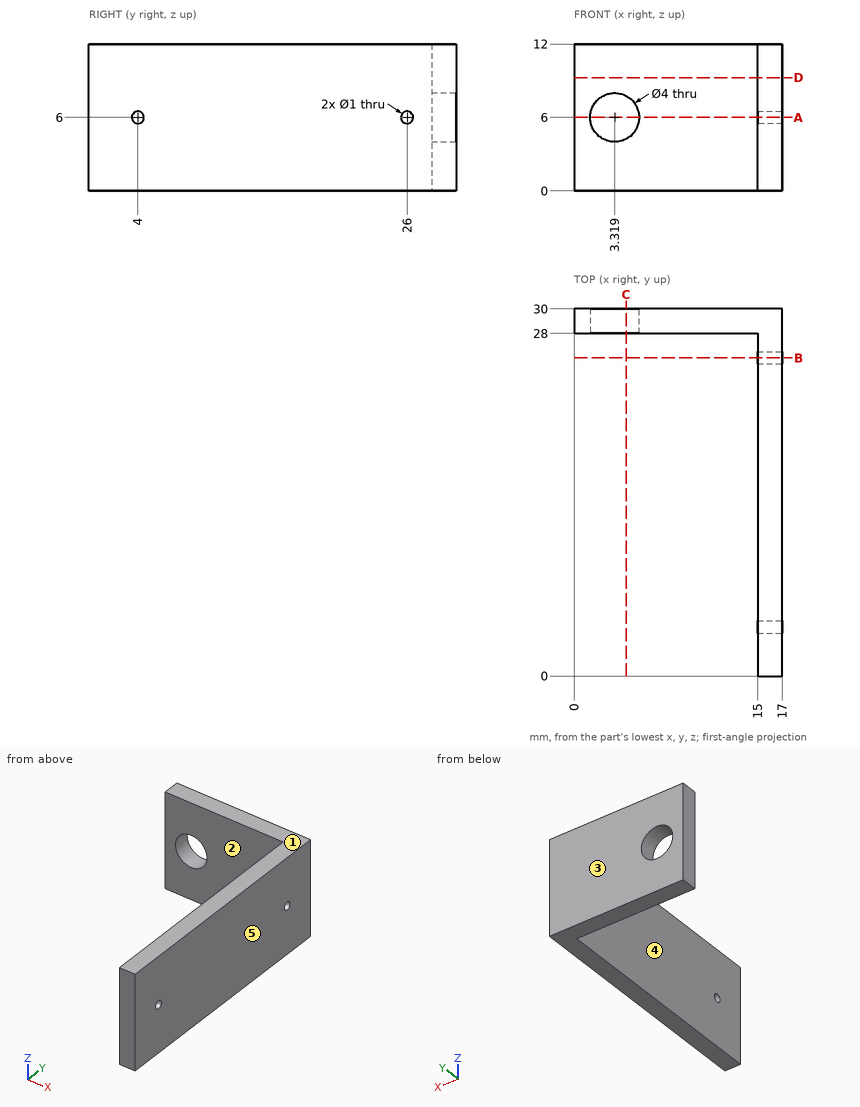
Geometry check sheet. Reference: drawing and pictorial views, mm from the part's lowest x, y, z. A direction names the side the tool comes from. Round coordinates to 2 decimals unless told otherwise and drop trailing zeros. Loops run counter-clockwise (first coordinate to the right, second up) from the corner with the lowest first, then second, coordinate; pieces in that order, holes last. Notation, with made-up numbers: (26.5, -37.75) - (78.5, -37.75) arc R27 cw to (78.5, -10.75) - close; hole circle Ø11 at (36.5, -0.5). An arc over 180 degrees is marked (long way). Answer as CSV lines item,"result".
(1) Material ranges on line 1 along Y through (x, z) = (16, 6); line 2 along Y through (x, z) = (10, 8.5); line 3 along X through (y, z) = (13.75, 2.75), recorded low to high.
Output values:
line 1,"y = 0 to 3.5, 4.5 to 25.5, 26.5 to 30"
line 2,"y = 28 to 30"
line 3,"x = 15 to 17"
(2) Release check for a two-part mould opening along Y. For the marked faces 1, 2 and 3 record: released by +Y, released by -Y, zero draft, split by the parting line, or undercut.
Output values:
face 1,"zero draft"
face 2,"released by -Y"
face 3,"released by +Y"
(3) Cross-section at B-B, the plane y = 26. Enter the section's corners in (x, z).
Output values:
outline,"(15, 0) - (17, 0) - (17, 5.5) - (15, 5.5) - close; (15, 6.5) - (17, 6.5) - (17, 12) - (15, 12) - close"
(4) Cross-section at D-D, the plane z = 9.25. Enter the section's corners in (x, y), and give its area (3 significant figures).
Output values:
outline,"(0, 28) - (15, 28) - (15, 0) - (17, 0) - (17, 30) - (0, 30) - close"
area,"90.0 mm²"
(5) Cross-section at A-A, the plane z = 6. Enter the section's corners in (x, y), and give its area (3 significant figures).
Output values:
outline,"(0, 28) - (1.32, 28) - (1.32, 30) - (0, 30) - close; (5.32, 28) - (15, 28) - (15, 26.5) - (17, 26.5) - (17, 30) - (5.32, 30) - close; (15, 0) - (17, 0) - (17, 3.5) - (15, 3.5) - close; (15, 4.5) - (17, 4.5) - (17, 25.5) - (15, 25.5) - close"
area,"78.0 mm²"
(6) Set-up check for the marked faces 4 and 5: record each of +Z, -Z, +X, -X, +Y, -Y from which the full face is reachable in a straight line by a thin tool's end or side.
Output values:
face 4,"+Z, -Z, -X, -Y"
face 5,"+Z, -Z, +X, +Y, -Y"
(7) Depth check by flat-ended pin: pin 1 Ø4 at (y, z) = (7, 9.5) entering from -X. Enter the tip coordinate at first touch or a pass-through.
Output values:
pin 1,"stops at x = 15"
(8) Cross-section at C-C, the plane x = 4.25. Enter the section's corners in (y, z).
Output values:
outline,"(28, 0) - (30, 0) - (30, 4.23) - (28, 4.23) - close; (28, 7.77) - (30, 7.77) - (30, 12) - (28, 12) - close"
